from build123d import *

# Parameters (mm, degrees)
SKETCH1_W           = 46
SKETCH1_H           = 36.614031046
BOSS_EXTRUDE1_DEPTH = 2.5
SKETCH2_W           = 2.5
SKETCH2_H           = 25.026075356
SKETCH2_H_2         = 7.18795569
BOSS_EXTRUDE2_DEPTH = 20.83511976
SKETCH4_W           = 10
SKETCH4_H           = 20.552854399
BOSS_EXTRUDE8_DEPTH = 5
SKETCH5_W           = 20.026075356
SKETCH5_H           = 23.33511976
CUT_EXTRUDE1_DEPTH  = 100
SKETCH6_W           = 49
SKETCH6_H           = 2.5
BOSS_EXTRUDE9_DEPTH = 44.601756686
SKETCH7_R           = 2.35
CUT_EXTRUDE2_DEPTH  = 57
SKETCH9_W           = 16.58795569
SKETCH9_H           = 2.782265361
CUT_EXTRUDE3_DEPTH  = 47
SKETCH10_R          = 1.5
CUT_EXTRUDE4_DEPTH  = 10


with BuildPart() as part:
    # Sketch1 → Boss-Extrude1 (new body)
    with BuildSketch(Plane(origin=(0, 0, 0), x_dir=(1, 0, 0), z_dir=(0, 1, 0))):
        with Locations((23, 18.307015523)):
            Rectangle(SKETCH1_W, SKETCH1_H)
    extrude(amount=BOSS_EXTRUDE1_DEPTH)

    # Sketch2 → Boss-Extrude2 (add)
    with BuildSketch(Plane(origin=(0, 2.5, 0), x_dir=(1, 0, 0), z_dir=(0, 1, 0))):
        with Locations((1.25, 24.100993368)):
            Rectangle(SKETCH2_W, SKETCH2_H)
        with Locations((1.25, 3.593977845)):
            Rectangle(SKETCH2_W, SKETCH2_H_2)
        with Locations((44.75, 3.593977845)):
            Rectangle(SKETCH2_W, SKETCH2_H_2)
        with Locations((44.75, 24.100993368)):
            Rectangle(SKETCH2_W, SKETCH2_H)
    extrude(amount=BOSS_EXTRUDE2_DEPTH)

    # Sketch4 → Boss-Extrude8 (add)
    with BuildSketch(Plane.XY.offset(-11.58795569)):
        with Locations((-2.5, 10.2764272)):
            Rectangle(SKETCH4_W, SKETCH4_H)
        with Locations((48.5, 10.2764272)):
            Rectangle(SKETCH4_W, SKETCH4_H)
    extrude(amount=-BOSS_EXTRUDE8_DEPTH)

    # Sketch5 → Cut-Extrude1 (cut)
    with BuildSketch(Plane.ZY):
        with Locations((-26.600993368, 11.66755988)):
            Rectangle(SKETCH5_W, SKETCH5_H)
    extrude(amount=-CUT_EXTRUDE1_DEPTH, mode=Mode.SUBTRACT)

    # Sketch6 → Boss-Extrude9 (add)
    with BuildSketch(Plane(origin=(0, 0, -16.58795569), x_dir=(-1, 0, 0), z_dir=(0, 0, -1))):
        with Locations((-23, 1.25)):
            Rectangle(SKETCH6_W, SKETCH6_H)
    extrude(amount=BOSS_EXTRUDE9_DEPTH)

    # Sketch7 → Cut-Extrude2 (cut)
    with BuildSketch(Plane(origin=(0, 2.5, 0), x_dir=(1, 0, 0), z_dir=(0, 1, 0))):
        with Locations(Location((4.458214718, 43.313777074, 0), (0, 0, 270))):
            Circle(SKETCH7_R)
        with Locations(Location((41.472783072, 43.313777074, 0), (0, 0, 270))):
            Circle(SKETCH7_R)
    extrude(amount=-CUT_EXTRUDE2_DEPTH, mode=Mode.SUBTRACT)

    # Sketch9 → Cut-Extrude3 (cut)
    with BuildSketch(Plane.ZY):
        with Locations((-8.293977845, 21.94398708)):
            Rectangle(SKETCH9_W, SKETCH9_H)
    extrude(amount=-CUT_EXTRUDE3_DEPTH, mode=Mode.SUBTRACT)

    # Sketch10 → Cut-Extrude4 (cut)
    with BuildSketch(Plane.XY.offset(-11.58795569)):
        with Locations((-1.353500868, 17.657737488)):
            Circle(SKETCH10_R)
        with Locations((-1.353500868, 7.492318257)):
            Circle(SKETCH10_R)
        with Locations((47.56068481, 17.657737488)):
            Circle(SKETCH10_R)
        with Locations((47.56068481, 7.492318257)):
            Circle(SKETCH10_R)
    extrude(amount=-CUT_EXTRUDE4_DEPTH, mode=Mode.SUBTRACT)


solid = part.part
Design review of the part built by this model. Coordinates are the model's own, in mm. A direction names the side the tool comes from. Round coordinates to 2 decimals unless told otherwise and drop trailing zeros. Write each loop counter-clockwise with the first axis right and the second up, starting at its lowest first coordinate (ties: lowest second). Pieces come first, ordered by that corner, then holes. Notation, with made-up numbers: (-24.5, -24.75) - (-16.5, -24.75) arc R29 cw to (-16.5, 6.25) - close; hole circle Ø3 at (-6, -12). An arc over 180 degrees is marked (long way). Use a Markdown table: item, result. Add a question column.
1. We need section B-B (z = -6). State the section outline as (x, y) points.
2. We need section C-C (x = 40). State the section outline as (y, z) points (3 decimals).
3. For faces 4 (the face through (47.5, 1, -39)), 5 (the face through (46, 10, -4)), 6 (the face through (-1.5, 1, -39)), 7 (the face through (45, 11, -7.188)), list the 3-axis set-ups (+Z, -Z, +X, -X, +Y, -Y) from which the entire face can be reached by the end or side of a thin tool; tool diameter is ignored.
4. Wall thickness on probe 1 along X at (y, z) = (13, -4); probe 2 along Z at (x, y) = (45, 11.5); probe 3 along X at (y, z) = (2.25, -45): over which ranges is each line inside the solid? List them lowest first.
5. We need section D-D (x = 24). State the section outline as (y, z) points.
6. Mouldability with a two-part tool opening along X and no side actions: class faces 1 (the face through (53.5, 10, -14)), 2 (the face through (23, 0, -30)), 3 (the face through (23, 2.5, -30)) as +X half, -X half, draft (parallel to the pull), parting line (faces both ways), or undercut.
7. We need section A-A (y = 10). State the section outline as (x, z) points.
8. Clearance check with flat-ended pins moving along their axes: pin 1 (1 mm diameter, centred on y = 7.5, z = -6, fed in from +X); pin 2 (0.8 mm diameter, centred on x = 44.5, y = 16, fed in from -Z); pin 3 (5.5 mm diameter, centred on x = 4.46, z = -43.31, fed in from +Y). State where each tip first meets the part, or that it passes through.
Output:
| question | item | result |
|---|---|---|
| 1 | outline | (0, 0) - (46, 0) - (46, 20.55) - (43.5, 20.55) - (43.5, 2.5) - (2.5, 2.5) - (2.5, 20.55) - (0, 20.55) - close |
| 2 | outline | (0, -61.19) - (2.5, -61.19) - (2.5, -45.145) - (0, -45.145) - close; (0, -41.483) - (2.5, -41.483) - (2.5, 0) - (0, 0) - close |
| 3 | face 4 | -Z, +X, +Y, -Y |
| 3 | face 5 | +Z, +X, +Y, -Y |
| 3 | face 6 | -Z, -X, +Y, -Y |
| 3 | face 7 | +X, -X, +Y |
| 4 | probe 1 | x = 0 to 2.5, 43.5 to 46 |
| 4 | probe 2 | z = -16.59 to -11.59, -7.19 to 0 |
| 4 | probe 3 | x = -1.5 to 2.82, 6.1 to 39.84, 43.11 to 47.5 |
| 5 | outline | (0, -61.19) - (2.5, -61.19) - (2.5, 0) - (0, 0) - close |
| 6 | face 1 | +X half |
| 6 | face 2 | draft |
| 6 | face 3 | undercut |
| 7 | outline | (-7.5, -16.59) - (2.5, -16.59) - (2.5, -11.59) - (-7.5, -11.59) - close; (0, -7.19) - (2.5, -7.19) - (2.5, 0) - (0, 0) - close; (43.5, -16.59) - (53.5, -16.59) - (53.5, -11.59) - (43.5, -11.59) - close; (43.5, -7.19) - (46, -7.19) - (46, 0) - (43.5, 0) - close |
| 8 | pin 1 | stops at x = 46 |
| 8 | pin 2 | stops at z = -16.59 |
| 8 | pin 3 | stops at y = 2.5 |
